Verification items for the finished model (mm, model axes). A direction names the side the tool comes from. Give positions to 0.01 mm unless a question says otherwise; leave off trailing zeros. Loops run counter-clockwise (first coordinate to the right, second up) from the corner with the lowest first, then second, coordinate; pieces in that order, holes last. Notation, with made-up numbers: M 4.5,-33 L 32.5,-33 A16 ccw 32.5,-16 Z; hole C 43.5,3.25 d7. An arc over 180 degrees is marked long. Answer in a Markdown table with one row per item.
```python
from build123d import *

# Parameters (mm, degrees)
BOSS_EXTRUDE1_DEPTH = 20.32
SKETCH3_W           = 23.583471357
SKETCH3_H           = 24.613240303
SKETCH3_H_2         = 23.081850847
SKETCH3_W_2         = 25.880555541
CUT_EXTRUDE1_DEPTH  = 120.044088604
SKETCH4_R           = 7.199159396
CUT_EXTRUDE2_DEPTH  = 147.168727436
SKETCH5_R           = 7.199159396
SKETCH5_R_2         = 7.039396065
CUT_EXTRUDE4_DEPTH  = 147.168727436


with BuildPart() as part:
    # Sketch2 → Boss-Extrude1 (new body)
    with BuildSketch(Plane(origin=(0, 0, 0), x_dir=(1, 0, 0), z_dir=(0, 1, 0))):
        with BuildLine():
            Line((-85.098911353, 55.935303266), (88.101088647, 55.935303266))
            ThreePointArc((88.101088647, 55.935303266), (98.707690365, 51.541904984), (103.101088647, 40.935303266))
            Line((103.101088647, 40.935303266), (103.101088647, -30.664696734))
            ThreePointArc((103.101088647, -30.664696734), (98.707690365, -41.271298452), (88.101088647, -45.664696734))
            Line((88.101088647, -45.664696734), (-85.098911353, -45.664696734))
            ThreePointArc((-85.098911353, -45.664696734), (-95.705513071, -41.271298452), (-100.098911353, -30.664696734))
            Line((-100.098911353, -30.664696734), (-100.098911353, 40.935303266))
            ThreePointArc((-100.098911353, 40.935303266), (-95.705513071, 51.541904984), (-85.098911353, 55.935303266))
        make_face()
    extrude(amount=-BOSS_EXTRUDE1_DEPTH)

    # Sketch3 → Cut-Extrude1 (cut, through all)
    with BuildSketch(Plane(origin=(0, 0, 0), x_dir=(1, 0, 0), z_dir=(0, 1, 0))):
        with Locations((99.892824326, 43.628683115)):
            Rectangle(SKETCH3_W, SKETCH3_H)
        with Locations((99.892824326, -34.123771311)):
            Rectangle(SKETCH3_W, SKETCH3_H_2)
        with Locations((-98.039189124, 43.628683115)):
            Rectangle(SKETCH3_W_2, SKETCH3_H)
        with Locations((-98.039189124, -34.123771311)):
            Rectangle(SKETCH3_W_2, SKETCH3_H_2)
    extrude(amount=-CUT_EXTRUDE1_DEPTH, mode=Mode.SUBTRACT)

    # Sketch4 → Cut-Extrude2 (cut, through all)
    with BuildSketch(Plane.XY.offset(45.664696734)):
        with Locations((54.410594351, -10.313138946)):
            Circle(SKETCH4_R)
    extrude(amount=-CUT_EXTRUDE2_DEPTH, mode=Mode.SUBTRACT)

    # Sketch5 → Cut-Extrude4 (cut, through all)
    with BuildSketch(Plane.XY.offset(45.664696734)):
        with Locations((54.410594351, -10.313138946)):
            Circle(SKETCH5_R)
        with Locations((-54.624334914, -10.313138946)):
            Circle(SKETCH5_R_2)
    extrude(amount=-CUT_EXTRUDE4_DEPTH, mode=Mode.SUBTRACT)


solid = part.part
```
Item 1: Tool access check on faces 1 (the flat face through (88.101, -10, -43)), 2 (the flat face through (-93, -10, 22.583)), 3 (the flat face through (88.101, -10, 34)), 4 (the flat face through (-85.099, -10, -43)). Record the directions out of +Z, -Z, +X, -X, +Y, -Y that give a thin tool (end or side, any length) a straight path to the whole face; none if there is none.
Reported:
| item | result |
|---|---|
| face 1 | -Z, +X, +Y, -Y |
| face 2 | +Z, -X, +Y, -Y |
| face 3 | +Z, +X, +Y, -Y |
| face 4 | -Z, -X, +Y, -Y |
Item 2: Go/stop test with flat-tipped pins: pin 1 (4.5 mm diameter, centred on x = 97.5, y = -12, fed in from -Z); pin 2 (7.5 mm diameter, centred on x = 93.5, y = -14.5, fed in from +Z). Record where each tip stops, or that it passes through.
Reported:
| item | result |
|---|---|
| pin 1 | stops at z = -31.32 |
| pin 2 | stops at z = 22.58 |
Item 3: Release check for a two-part mould opening along X. For faces 5 (the flat face through (-100.099, -10, -4)), 6 (the flat face through (95, -10, -31.322)), 7 (the cylindrical face through (-61.657, -10.004, -4.424)) record: released by +X, released by -X, zero draft, split by the parting line, or undercut.
Reported:
| item | result |
|---|---|
| face 5 | released by -X |
| face 6 | zero draft |
| face 7 | undercut |
Item 4: Scan lines: L1, parallel to X at y = -9.75, z = 38.5; L2, parallel to Y at x = -54, z = -13; L3, parallel to X at y = -7, z = 39. Record each from-to range of solid material in increasing order. Write a range as [from, to].
Reported:
| item | result |
|---|---|
| L1 | x = [-85.1, -61.64], [-47.61, 47.23], [61.59, 88.1] |
| L2 | y = [-20.32, -17.32], [-3.3, 0] |
| L3 | x = [-85.1, -60.84], [-48.41, 48.02], [60.8, 88.1] |
Item 5: Sectioned sample at B-B (x = 51.5). Record the cut outline in (y, z).
Reported:
| item | result |
|---|---|
| outline | M -20.32,-55.94 L -16.9,-55.94 L -16.9,45.66 L -20.32,45.66 Z; M -3.73,-55.94 L 0,-55.94 L 0,45.66 L -3.73,45.66 Z |
Item 6: Sectioned sample at A-A (y = -8). Record the cut outline in (x, z), and give its area (3 significant figures).
Reported:
| item | result |
|---|---|
| outline | M -100.1,-31.32 L -85.1,-31.32 L -85.1,-55.94 L -61.27,-55.94 L -61.27,45.66 L -85.1,45.66 L -85.1,22.58 L -100.1,22.58 Z; M -47.98,-55.94 L 47.59,-55.94 L 47.59,45.66 L -47.98,45.66 Z; M 61.23,-55.94 L 88.1,-55.94 L 88.1,-31.32 L 103.1,-31.32 L 103.1,22.58 L 88.1,22.58 L 88.1,45.66 L 61.23,45.66 Z |
| area | 16,500 mm^2 |
Item 7: Sectioned sample at D-D (x = -56.5). Record the cut outline in (y, z), and give its area (3 significant figures).
Reported:
| item | result |
|---|---|
| outline | M -20.32,-55.94 L -17.1,-55.94 L -17.1,45.66 L -20.32,45.66 Z; M -3.53,-55.94 L 0,-55.94 L 0,45.66 L -3.53,45.66 Z |
| area | 686 mm^2 |
Item 8: Sectioned sample at C-C (z = 24.5). Record the cut outline in (x, y).
Reported:
| item | result |
|---|---|
| outline | M -85.1,-20.32 L 88.1,-20.32 L 88.1,0 L -85.1,0 Z; hole C -54.62,-10.31 d14.08; hole C 54.41,-10.31 d14.4 |
